The listing builds one solid part. Answer for the finished solid, in the listing's coordinates (mm). Face numbers are marked on the shaded views. A direction names the side the tool comes from. Round coordinates to 2 decimals unless told otherwise and drop trailing zeros. Write each loop counter-clockwise with the first axis right and the second up, starting at its lowest first coordinate (ties: lowest second). Pieces come first, ordered by that corner, then holes.
Item 1: Each of these flat-tipped pins is pushed along its axis until it touches: pin 1 (2 mm diameter, centred on x = -0.5, z = -2.5, fed in from +Y); pin 2 (6 mm diameter, centred on x = -4.5, y = 3.5, fed in from -Z); pin 3 (2 mm diameter, centred on y = -2.5, z = 4.5, fed in from +X); pin 4 (2 mm diameter, centred on x = 1.5, y = -3, fed in from -Z). Where does it stop, or does it pass through?
Item 2: Find section C-C on y = -2. Give the vertices of the cut face in (x, z), then the cut area to 3 significant figures.
Item 3: Find section A-A on z = 0. Give the vertices of the cut face in (x, y).
Item 4: For a pull along X with two mould halves and no side action, classify the marked faces 1, 2 and 3 as +X half, -X half, draft (parallel to the pull), parting line (faces both ways), or undercut.
Item 5: Find section B-B on x = 0. Give the vertices of the cut face in (y, z).
Item 6: A tool of negligible diameter and unlimited length cuts with its end or side. For the marked faces 4 and 5, from which of +Z, -Z, +X, -X, +Y, -Y can it reach the whole face along a straight path? Write none if from no direction.
Item 7: Find the intervals of material crossed by probe 1 along Z at (x, y) = (1.5, 2.25); probe 2 along X at (y, z) = (-1, 3.5); probe 3 along X at (y, z) = (0, 8.05), in increasing order.
```python
from build123d import *

# Parameters (mm, degrees)
F0_R     = 9
F0_R_2   = 4.5
F1_DEPTH = 5
F2_R     = 1.5
F3_DEPTH = 9.001
F4_SIZE  = 1


with BuildPart() as f1:
    # F0 (on Front) → F1 (new body, symmetric)
    with BuildSketch(Plane.XZ):
        Circle(F0_R)
        Circle(F0_R_2, mode=Mode.SUBTRACT)
    extrude(amount=F1_DEPTH, both=True)

    # F2 (on Top) → F3 (cut, through all)
    with BuildSketch(Plane.XY):
        Circle(F2_R)
    extrude(amount=F3_DEPTH, mode=Mode.SUBTRACT)

    # F4
    f4_edges = [f1.edges().sort_by_distance(p)[0] for p in [
        (-9, -5, 0),
        (-9, 5, 0),
    ]]
    chamfer(f4_edges, length=F4_SIZE)


solid = f1.part
```
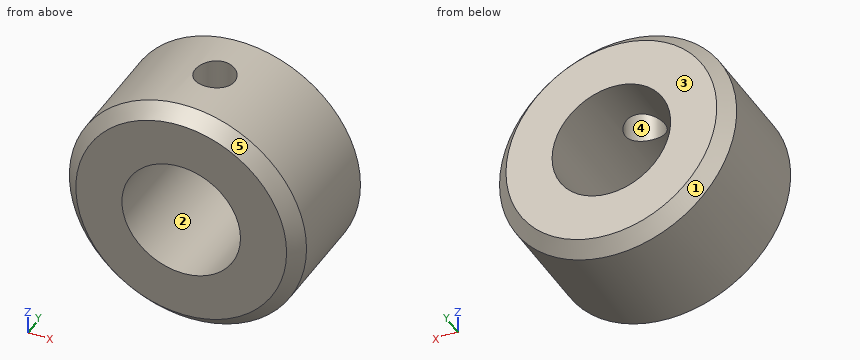
Check values:
1. pin 1: passes through
1. pin 2: stops at z = -8.87
1. pin 3: stops at x = 8.29
1. pin 4: stops at z = -8.99
2. outline: circle Ø18 at (0, 0); hole circle Ø9 at (0, 0)
2. area: 191 mm2
3. outline: (-9, -4) - (-8, -5) - (-4.5, -5) - (-4.5, 5) - (-8, 5) - (-9, 4) - close; (4.5, -5) - (8, -5) - (9, -4) - (9, 4) - (8, 5) - (4.5, 5) - close
4. face 1: parting line
4. face 2: undercut
4. face 3: draft
5. outline: (-5, -8) - (-4, -9) - (4, -9) - (5, -8) - (5, -4.5) - (-5, -4.5) - close; (-5, 4.5) - (-1.5, 4.5) - (-1.5, 9) - (-4, 9) - (-5, 8) - close; (1.5, 4.5) - (5, 4.5) - (5, 8) - (4, 9) - (1.5, 9) - close
6. face 4: +Z
6. face 5: -Y
7. probe 1: z = -8.87 to -4.24, 4.24 to 8.87
7. probe 2: x = -8.29 to -2.83, 2.83 to 8.29
7. probe 3: x = -4.02 to -1.5, 1.5 to 4.02
